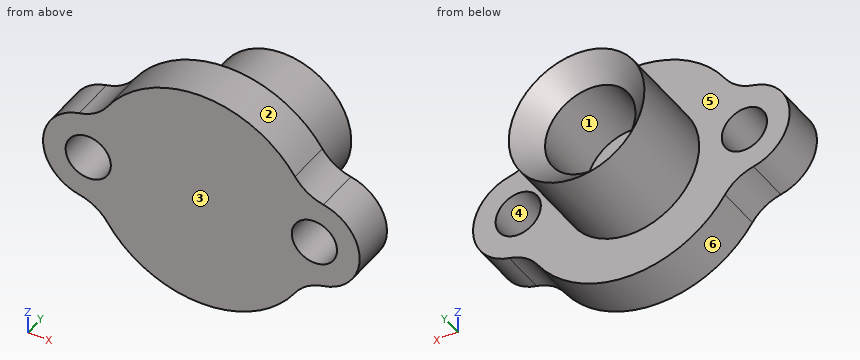
from build123d import *

# Parameters (mm, degrees)
SKETCH1_R           = 5
BOSS_EXTRUDE1_DEPTH = 10
SKETCH2_R           = 15
SKETCH2_R_2         = 10
BOSS_EXTRUDE2_DEPTH = 25
CHAMFER2_SIZE       = 10


with BuildPart() as part:
    # Sketch1 → Boss-Extrude1 (new body)
    with BuildSketch(Plane(origin=(0, 0, 0), x_dir=(1, 0, 0), z_dir=(0, 1, 0))):
        with BuildLine():
            ThreePointArc((-20.714285714, -13.997084244), (0, -25), (20.714285714, -13.997084244))
            ThreePointArc((20.714285714, -13.997084244), (23.445079401, -11.280699536), (27, -9.797958971))
            ThreePointArc((27, -9.797958971), (35, 0), (27, 9.797958971))
            ThreePointArc((27, 9.797958971), (23.445079401, 11.280699536), (20.714285714, 13.997084244))
            ThreePointArc((20.714285714, 13.997084244), (0, 25), (-20.714285714, 13.997084244))
            ThreePointArc((-20.714285714, 13.997084244), (-23.445079401, 11.280699536), (-27, 9.797958971))
            ThreePointArc((-27, 9.797958971), (-35, 0), (-27, -9.797958971))
            ThreePointArc((-27, -9.797958971), (-23.445079401, -11.280699536), (-20.714285714, -13.997084244))
        make_face()
        with Locations(Location((25, 0, 0), (0, 0, 270))):
            Circle(SKETCH1_R, mode=Mode.SUBTRACT)
        with Locations(Location((-25, 0, 0), (0, 0, 90))):
            Circle(SKETCH1_R, mode=Mode.SUBTRACT)
    extrude(amount=BOSS_EXTRUDE1_DEPTH)

    # Sketch2 → Boss-Extrude2 (add)
    with BuildSketch(Plane(origin=(0, 10, 0), x_dir=(1, 0, 0), z_dir=(0, 1, 0))):
        with Locations(Location((0, 0, 0), (0, 0, 270))):
            Circle(SKETCH2_R)
        with Locations(Location((0, 0, 0), (0, 0, 270))):
            Circle(SKETCH2_R_2, mode=Mode.SUBTRACT)
    extrude(amount=BOSS_EXTRUDE2_DEPTH)

    # Chamfer2
    # the kernel refuses this chamfer: 10 mm, written as the material it takes off along each edge
    with BuildSketch(Plane(origin=(0, 35, 0), x_dir=(0, 0, 1), z_dir=(-1, 0, 0))) as chamfer2_piece_1:
        Polygon((10 + CHAMFER2_SIZE, 0), (10, -CHAMFER2_SIZE), (10, 0), align=None)
    revolve(axis=Axis((0, 35, 0), (0, 1, 0)), mode=Mode.SUBTRACT)


solid = part.part
Check sheet for the modelled part. Datum: model origin and axes. Units: mm. Face numbers are marked on the shaded views. A direction names the side the tool comes from. Give positions to 0.01 mm unless a question says otherwise; leave off trailing zeros. Write each loop counter-clockwise with the first axis right and the second up, starting at its lowest first coordinate (ties: lowest second). Pieces come first, ordered by that corner, then holes. Notation, with made-up numbers: M -15.75,42.25 L 21.25,42.25 A10 cw 21.25,51.25 Z; hole C 89.25,-27 d6. An arc over 180 degrees is marked long. Use one line per item in the form item = value.
(1) Depth check by flat-ended pin: P1, Ø10, axis at x = 26.5, z = 1, coming from the +Y side; P2, Ø1, axis at x = 25, z = 9, coming from the -Y side; P3, Ø3, axis at y = 13, z = 1, coming from the -X side; P4, Ø10, axis at x = -5.5, y = 21.5, coming from the +Z side. Enter the tip coordinate at first touch or a pass-through.
Answer block:
P1 = 10
P2 = 0
P3 = -15
P4 = 14.99
(2) Section check C-C on x = 0. Record the boundary of the cut face in (y, z).
Answer block:
outline = M 0,-25 L 10,-25 L 10,-15 L 30,-15 L 25,-10 L 10,-10 L 10,10 L 25,10 L 30,15 L 10,15 L 10,25 L 0,25 Z
(3) Section check B-B on x = -25. Record the boundary of the cut face in (y, z), plus the area to 3 significant figures.
Answer block:
outline = M 0,-10.43 L 10,-10.43 L 10,-5 L 0,-5 Z; M 0,5 L 10,5 L 10,10.43 L 0,10.43 Z
area = 109 mm2
(4) Tool access check on the marked faces 5 and 6. Record the directions out of +Z, -Z, +X, -X, +Y, -Y that give a thin tool (end or side, any length) a straight path to the whole face; none if there is none.
Answer block:
face_5 = +Y
face_6 = -Z, +Y, -Y
(5) Section check A-A on z = 0. Record the boundary of the cut face in (x, y), plus the area to 3 significant figures.
Answer block:
outline = M -35,0 L -30,0 L -30,10 L -35,10 Z; M -20,0 L 20,0 L 20,10 L 15,10 L 15,30 L 10,25 L 10,10 L -10,10 L -10,25 L -15,30 L -15,10 L -20,10 Z; M 30,0 L 35,0 L 35,10 L 30,10 Z
area = 675 mm2
(6) Material ranges on line 1 along X through (y, z) = (24.75, -0.5); line 2 along Z through (x, y) = (-4, 20); line 3 along X through (y, z) = (24, 1), recorded low to high.
Answer block:
line_1 = -14.99 to -9.99, 9.99 to 14.99
line_2 = -14.46 to -9.17, 9.17 to 14.46
line_3 = -14.97 to -9.95, 9.95 to 14.97
(7) Section check D-D on y = 16.75. Record the boundary of the cut face in (x, z), plus the area to 3 significant figures.
Answer block:
outline = C 0,0 d30; hole C 0,0 d20
area = 393 mm2
(8) Draft check along Z on the marked faces 1, 2, 3 and 4. Enter one of: pulls with the +Z half, pulls with the -Z half, needs draft (parallel to the pull), parting line crosses it, or undercut.
Answer block:
face_1 = undercut
face_2 = pulls with the +Z half
face_3 = needs draft
face_4 = undercut
